Here's how the part is built. I have some questions about the finished solid (model axes, mm). Give positions to 0.01 mm unless a question says otherwise; leave off trailing zeros. Use a Markdown table: item, result.
from build123d import *

# Parameters (mm, degrees)
SKETCH1_W            = 152.20001
SKETCH1_H            = 134.65
BOSS_EXTRUDE1_DEPTH  = 12.5
M8_CLEARANCE_HOLE1_D = 9
M8_CLEARANCE_HOLE2_D = 9
FILLET1_R            = 10
CUT_EXTRUDE1_DEPTH   = 10.5
CUT_EXTRUDE2_DEPTH   = 7.5
CUT_EXTRUDE3_START   = -12.5
CUT_EXTRUDE3_DEPTH   = 6


with BuildPart() as part:
    # Sketch1 → Boss-Extrude1 (new body)
    with BuildSketch(Plane(origin=(0, 0, 0), x_dir=(1, 0, 0), z_dir=(0, 1, 0))):
        with Locations((50.699995, 42.325)):
            Rectangle(SKETCH1_W, SKETCH1_H)
    extrude(amount=BOSS_EXTRUDE1_DEPTH)

    # M8 Clearance Hole1 (through all)
    with Locations(Plane(origin=(0, 0, 0), x_dir=(-1, 0, 0), z_dir=(0, -1, 0))):
        with Locations((-102.19999, 42.11), (0.40001, 42.11), (0.40001, 98.26), (-102.19999, 98.26)):
            Hole(M8_CLEARANCE_HOLE1_D / 2)

    # M8 Clearance Hole2 (through all)
    with Locations(Plane(origin=(0, 0, 0), x_dir=(-1, 0, 0), z_dir=(0, -1, 0))):
        with Locations((-101.8, 0), (0, 0), (-101.8, 79.65), (0, 79.65)):
            Hole(M8_CLEARANCE_HOLE2_D / 2)

    # Fillet1
    fillet1_edges = [part.edges().sort_by_distance(p)[0] for p in [
        (-25.40001, 6.25, -109.65),
        (126.8, 6.25, -109.65),
        (126.8, 6.25, 25),
        (-25.40001, 6.25, 25),
    ]]
    fillet(fillet1_edges, radius=FILLET1_R)

    # Sketch12 → Cut-Extrude1 (cut)
    with BuildSketch(Plane(origin=(0, 12.5, 0), x_dir=(1, 0, 0), z_dir=(0, 1, 0))):
        Polygon((94.294446501, 79.65), (98.04722325, 73.15), (105.55277675, 73.15), (109.305553499, 79.65), (105.55277675, 86.15), (98.04722325, 86.15), align=None)
        Polygon((94.294446501, 0), (98.04722325, -6.5), (105.55277675, -6.5), (109.305553499, 0), (105.55277675, 6.5), (98.04722325, 6.5), align=None)
    extrude(amount=-CUT_EXTRUDE1_DEPTH, mode=Mode.SUBTRACT)

    # Sketch12<4> → Cut-Extrude2 (cut)
    with BuildSketch(Plane(origin=(0, 12.5, 0), x_dir=(1, 0, 0), z_dir=(0, 1, 0))):
        Polygon((7.505553499, 79.65), (3.75277675, 86.15), (-3.75277675, 86.15), (-7.505553499, 79.65), (-3.75277675, 73.15), (3.75277675, 73.15), align=None)
        Polygon((7.505553499, 0), (3.75277675, 6.5), (-3.75277675, 6.5), (-7.505553499, 0), (-3.75277675, -6.5), (3.75277675, -6.5), align=None)
    extrude(amount=-CUT_EXTRUDE2_DEPTH, mode=Mode.SUBTRACT)

    # Sketch12<5> → Cut-Extrude3 (cut)
    with BuildSketch(Plane(origin=(0, 12.5, 0), x_dir=(1, 0, 0), z_dir=(0, 1, 0)).offset(CUT_EXTRUDE3_START)):
        Polygon((7.105543499, 98.26), (3.35276675, 104.76), (-4.15278675, 104.76), (-7.905563499, 98.26), (-4.15278675, 91.76), (3.35276675, 91.76), align=None)
        Polygon((109.705543499, 98.26), (105.95276675, 104.76), (98.44721325, 104.76), (94.694436501, 98.26), (98.44721325, 91.76), (105.95276675, 91.76), align=None)
        Polygon((7.105543499, 42.11), (3.35276675, 48.61), (-4.15278675, 48.61), (-7.905563499, 42.11), (-4.15278675, 35.61), (3.35276675, 35.61), align=None)
        Polygon((109.705543499, 42.11), (105.95276675, 48.61), (98.44721325, 48.61), (94.694436501, 42.11), (98.44721325, 35.61), (105.95276675, 35.61), align=None)
    extrude(amount=CUT_EXTRUDE3_DEPTH, mode=Mode.SUBTRACT)


solid = part.part
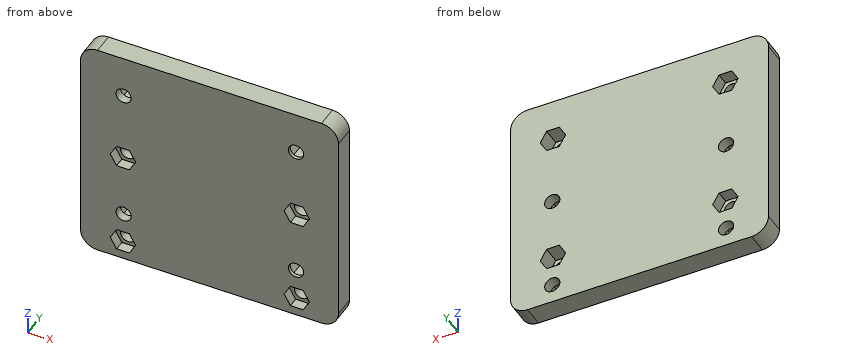
(1) If I drill on line 1 (X direction, y = 11, z = -42.11); line 2 (X direction, y = 1, z = -79.65); line 3 (Z direction, x = 0, y = 1.35), over which ranges is the centre line in solid material (lowest first)?
A:
| item | result |
|---|---|
| line 1 | -25.4 to -4.9, 4.1 to 97.7, 106.7 to 126.8 |
| line 2 | -25.4 to -4.5, 4.5 to 97.3, 106.3 to 126.8 |
| line 3 | -109.65 to -104.76, -91.76 to -84.15, -75.15 to -48.61, -35.61 to -4.5, 4.5 to 25 |
(2) Suppose I cut it at A-A on x = 101.8. Count the separate pieces of the cut face and the enclosed holes in it, plus the area to 3 significant figures.
A:
| item | result |
|---|---|
| separate pieces | 5 |
| enclosed holes | 0 |
| area | 1,100 mm2 |
(3) Will this pin go through, and if not, where does the flat tip stop? pin 1 (11.5 mm diameter, centred on x = 101.8, z = 0, fed in from +Y).
A:
| item | result |
|---|---|
| pin 1 | y = 2 |
